For this review, use the dimensioned drawing (mm, ordinates from the lowest corner) and the shaded views. Give positions to 0.01 mm unless a question says otherwise; leave off trailing zeros. Loops run counter-clockwise (first coordinate to the right, second up) from the corner with the lowest first, then second, coordinate; pieces in that order, holes last. Notation, with made-up numbers: M 49.25,-39 L 100.25,-39 A28 ccw 100.25,-4 Z; hole C 36.5,42 d1. An arc over 180 degrees is marked long. Return JSON: item names as keys, results as strings.
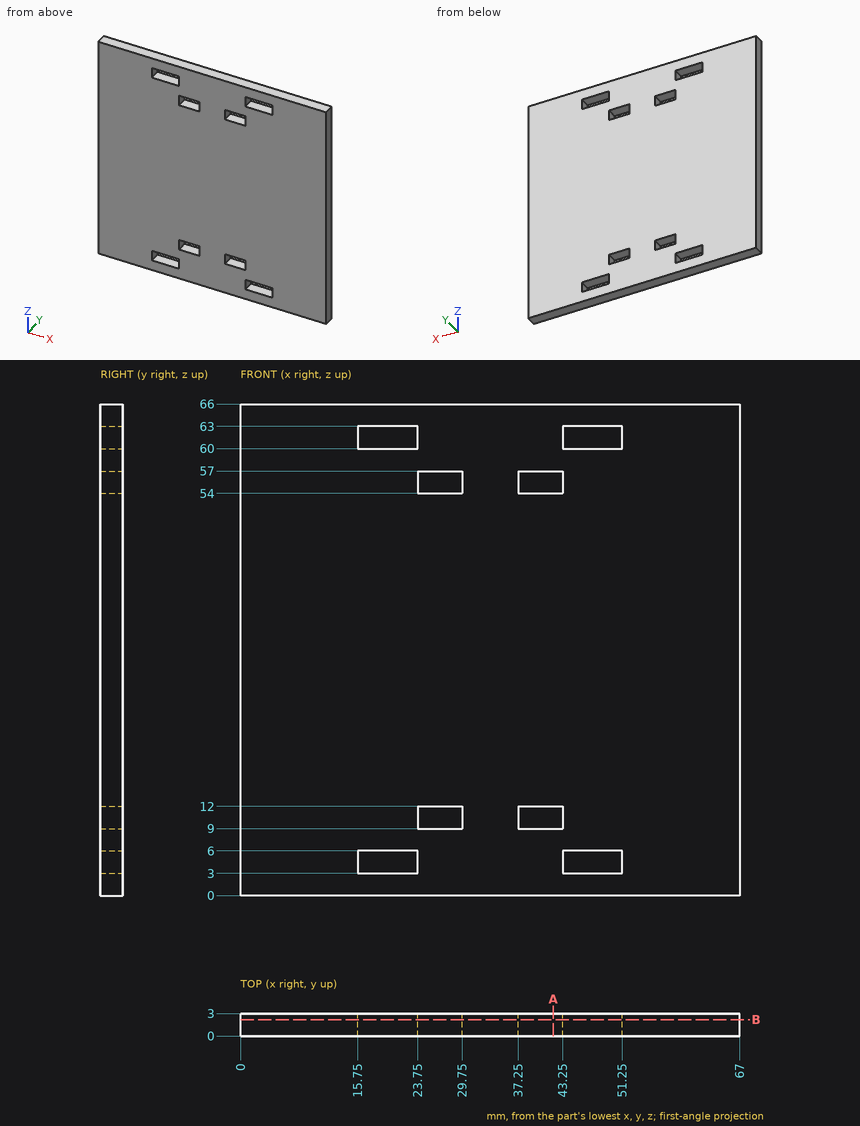
1) Consider section A-A on x = 42. Write out the cut boundary in (y, z), then the cut area to 3 significant figures.
From the geometry:
{"outline": "M 0,0 L 3,0 L 3,9 L 0,9 Z; M 0,12 L 3,12 L 3,54 L 0,54 Z; M 0,57 L 3,57 L 3,66 L 0,66 Z", "area": "180 mm²"}
2) Consider section B-B on y = 2.2. Count the separate pieces of the cut face and the enclosed holes in it, then the cut area to 3 significant figures.
From the geometry:
{"separate pieces": "1", "enclosed holes": "8", "area": "4,250 mm²"}
3) Wall thickness on L1, parallel to Z at x = 24, y = 0.2; L2, parallel to Z at x = 49.5, y = 2.55: over which ranges is each line inside the solid? List them lowest first. Write a range as from..to.
From the geometry:
{"L1": "0..9, 12..54, 57..66", "L2": "0..3, 6..60, 63..66"}
